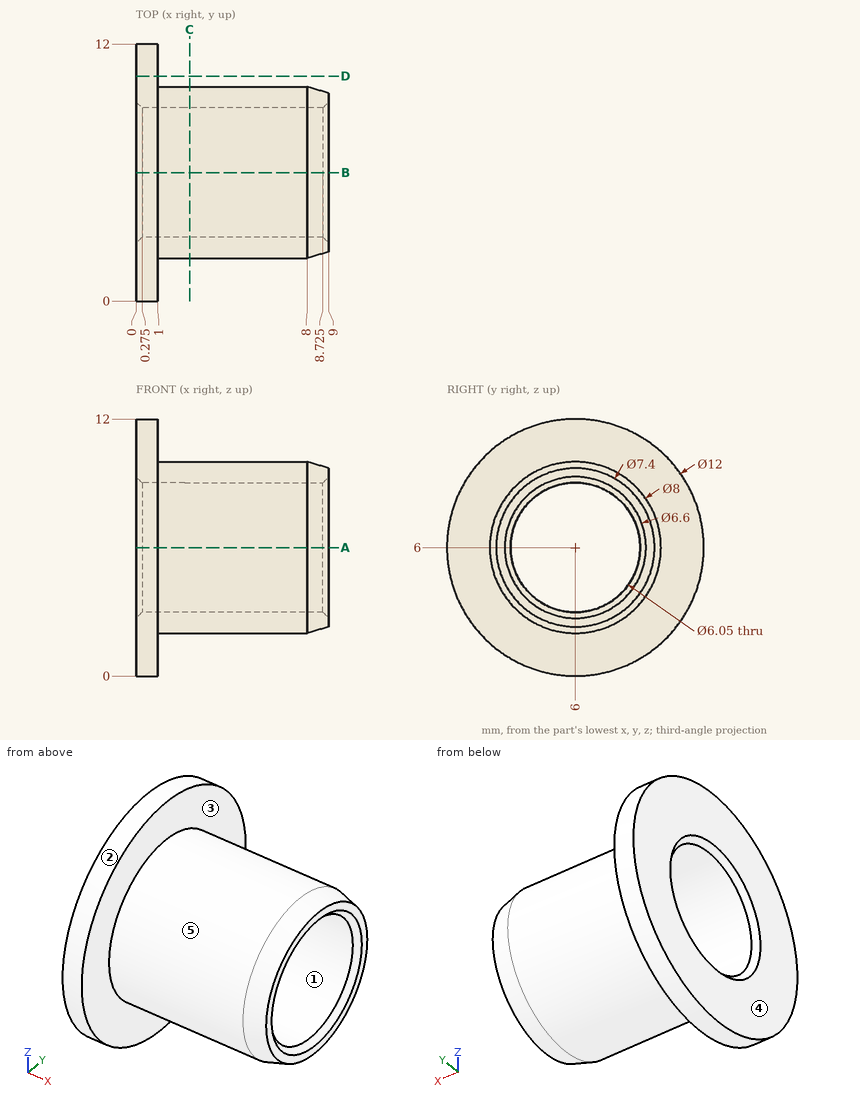
Drawing for the job (mm, zero at the part's lowest x, y, z). A direction names the side the tool comes from. Give positions to 0.01 mm unless a question says otherwise; leave off trailing zeros. Loops run counter-clockwise (first coordinate to the right, second up) from the corner with the lowest first, then second, coordinate; pieces in that order, holes last.
Item 1: Slice it at C-C (x = 2.5). Write the cut outline in (y, z) (3 decimals).
Check values:
outline: circle Ø8 at (6, 6); hole circle Ø6.05 at (6, 6)
Item 2: Drop flat-ended pins along their axis: P1, Ø3, axis at x = 8, z = 7.5, coming from the -Y side; P2, Ø2, axis at x = 3.5, z = 2.5, coming from the +Y side. Give the stop position or say it passes through.
Check values:
P1: stops at y = 2
P2: stops at y = 9.12
Item 3: Which spindle directions (+Z, -Z, +X, -X, +Y, -Y) get a long thin tool onto all of the face, cutting with end or side? Do the marked faces 4 and 5. Say none if no direction does.
Check values:
face 4: +Z, -Z, -X, +Y, -Y
face 5: +X
Item 4: Mould opens along Y. For the marked faces 1, 2 and 3 say: +Y half, -Y half, draft (parallel to the pull), parting line (faces both ways), or undercut.
Check values:
face 1: undercut
face 2: parting line
face 3: draft
Item 5: Slice it at A-A (z = 6). Write the cut outline in (x, y) (3 decimals), plus the area to 3 significant figures.
Check values:
outline: (0, 0) - (1, 0) - (1, 2) - (8, 2) - (9, 2.3) - (9, 2.7) - (8.725, 2.975) - (0.275, 2.975) - (0, 2.7) - close; (0, 9.3) - (0.275, 9.025) - (8.725, 9.025) - (9, 9.3) - (9, 9.7) - (8, 10) - (1, 10) - (1, 12) - (0, 12) - close
area: 21.1 mm2
Item 6: Drill centre lines: line 1 along Z through (x, y) = (2, 6) (3 decimals); line 2 along X through (y, z) = (10.25, 6.5); line 3 along Z through (x, y) = (5, 5.25). Where is each one in solid material? Low to high.
Check values:
line 1: z = 2 to 2.975, 9.025 to 10
line 2: x = 0 to 1
line 3: z = 2.07 to 3.07, 8.93 to 9.93
Item 7: Slice it at D-D (y = 10.5). Write the cut outline in (x, z).
Check values:
outline: (0, 2.03) - (1, 2.03) - (1, 9.97) - (0, 9.97) - close
